Work out the finished part from the listing and answer in its coordinate system (mm). A direction names the side the tool comes from. Round coordinates to 2 decimals unless told otherwise and drop trailing zeros. Loops run counter-clockwise (first coordinate to the right, second up) from the corner with the lowest first, then second, coordinate; pieces in that order, holes last.
```python
from build123d import *

# Parameters (mm, degrees)
SKETCH1_W           = 8.89
SKETCH1_H           = 8.89
BOSS_EXTRUDE1_DEPTH = 5.334
SKETCH2_W           = 1.524
SKETCH2_H           = 8.89
CUT_EXTRUDE1_DEPTH  = 3.302
FILLET3_RADIUS      = 0.3683
FILLET3_LENGTH      = 8.89
FILLET4_RADIUS      = 0.254
FILLET4_LENGTH      = 8.89
FILLET5_RADIUS      = 0.254
FILLET5_LENGTH      = 8.89
FILLET6_RADIUS      = 0.254
FILLET6_LENGTH      = 8.89
FILLET7_RADIUS      = 0.2667
FILLET7_LENGTH      = 8.89


with BuildPart() as part:
    # Sketch1 → Boss-Extrude1 (new body)
    with BuildSketch(Plane(origin=(0, 0, 0), x_dir=(1, 0, 0), z_dir=(0, 1, 0))):
        Rectangle(SKETCH1_W, SKETCH1_H)
    extrude(amount=BOSS_EXTRUDE1_DEPTH)

    # Sketch2 → Cut-Extrude1 (cut)
    with BuildSketch(Plane(origin=(0, 5.334, 0), x_dir=(1, 0, 0), z_dir=(0, 1, 0))):
        with Locations((-3.1496, 0)):
            Rectangle(SKETCH2_W, SKETCH2_H)
        with Locations((-1.1176, 0)):
            Rectangle(SKETCH2_W, SKETCH2_H)
        with Locations((0.9144, 0)):
            Rectangle(SKETCH2_W, SKETCH2_H)
        with Locations((2.9464, 0)):
            Rectangle(SKETCH2_W, SKETCH2_H)
    extrude(amount=-CUT_EXTRUDE1_DEPTH, mode=Mode.SUBTRACT)

    # Fillet3: full round fillet: the end face becomes a half cylinder, R = half its width
    fillet3_face = Plane((4.0767, 5.334, 0), x_dir=(0, 0, -1), z_dir=(0, 1, 0))  # on the end face: x along it, z out of the body
    fillet3_slab = fillet3_face.offset(-FILLET3_RADIUS / 2) * Box(FILLET3_LENGTH, 2 * FILLET3_RADIUS, FILLET3_RADIUS, mode=Mode.PRIVATE)  # the body's end, R deep
    fillet3_round = Plane((4.0767, 4.9657, 0), x_dir=(0, 1, 0), z_dir=(0, 0, -1)) * Cylinder(FILLET3_RADIUS, FILLET3_LENGTH, mode=Mode.PRIVATE)  # its axis R under the face
    add(fillet3_slab - fillet3_round, mode=Mode.SUBTRACT)

    # Fillet4: full round fillet: the end face becomes a half cylinder, R = half its width
    fillet4_face = Plane((1.9304, 5.334, 0), x_dir=(0, 0, 1), z_dir=(0, 1, 0))  # on the end face: x along it, z out of the body
    fillet4_slab = fillet4_face.offset(-FILLET4_RADIUS / 2) * Box(FILLET4_LENGTH, 2 * FILLET4_RADIUS, FILLET4_RADIUS, mode=Mode.PRIVATE)  # the body's end, R deep
    fillet4_round = Plane((1.9304, 5.08, 0), x_dir=(0, 1, 0), z_dir=(0, 0, 1)) * Cylinder(FILLET4_RADIUS, FILLET4_LENGTH, mode=Mode.PRIVATE)  # its axis R under the face
    add(fillet4_slab - fillet4_round, mode=Mode.SUBTRACT)

    # Fillet5: full round fillet: the end face becomes a half cylinder, R = half its width
    fillet5_face = Plane((-0.1016, 5.334, 0), x_dir=(0, 0, 1), z_dir=(0, 1, 0))  # on the end face: x along it, z out of the body
    fillet5_slab = fillet5_face.offset(-FILLET5_RADIUS / 2) * Box(FILLET5_LENGTH, 2 * FILLET5_RADIUS, FILLET5_RADIUS, mode=Mode.PRIVATE)  # the body's end, R deep
    fillet5_round = Plane((-0.1016, 5.08, 0), x_dir=(0, 1, 0), z_dir=(0, 0, 1)) * Cylinder(FILLET5_RADIUS, FILLET5_LENGTH, mode=Mode.PRIVATE)  # its axis R under the face
    add(fillet5_slab - fillet5_round, mode=Mode.SUBTRACT)

    # Fillet6: full round fillet: the end face becomes a half cylinder, R = half its width
    fillet6_face = Plane((-2.1336, 5.334, 0), x_dir=(0, 0, 1), z_dir=(0, 1, 0))  # on the end face: x along it, z out of the body
    fillet6_slab = fillet6_face.offset(-FILLET6_RADIUS / 2) * Box(FILLET6_LENGTH, 2 * FILLET6_RADIUS, FILLET6_RADIUS, mode=Mode.PRIVATE)  # the body's end, R deep
    fillet6_round = Plane((-2.1336, 5.08, 0), x_dir=(0, 1, 0), z_dir=(0, 0, 1)) * Cylinder(FILLET6_RADIUS, FILLET6_LENGTH, mode=Mode.PRIVATE)  # its axis R under the face
    add(fillet6_slab - fillet6_round, mode=Mode.SUBTRACT)

    # Fillet7: full round fillet: the end face becomes a half cylinder, R = half its width
    fillet7_face = Plane((-4.1783, 5.334, 0), x_dir=(0, 0, 1), z_dir=(0, 1, 0))  # on the end face: x along it, z out of the body
    fillet7_slab = fillet7_face.offset(-FILLET7_RADIUS / 2) * Box(FILLET7_LENGTH, 2 * FILLET7_RADIUS, FILLET7_RADIUS, mode=Mode.PRIVATE)  # the body's end, R deep
    fillet7_round = Plane((-4.1783, 5.0673, 0), x_dir=(0, 1, 0), z_dir=(0, 0, 1)) * Cylinder(FILLET7_RADIUS, FILLET7_LENGTH, mode=Mode.PRIVATE)  # its axis R under the face
    add(fillet7_slab - fillet7_round, mode=Mode.SUBTRACT)


solid = part.part
```
1. Which of the six approach directions +Z, -Z, +X, -X, +Y, -Y give full straight-line access (tool end or side, diameter ignored) to faces 4 (the face through (-3.912, 4, 0)), 5 (the face through (0, 2, -4.445))?
Answer key:
face 4: +Z, -Z, +Y
face 5: -Z, +X, -X, +Y, -Y
2. Find section A-A (z = -1.25). Write down the section's boundary in (x, y) (3 decimals), then the cut area to 3 significant figures.
Answer key:
outline: (-4.445, 0) - (4.445, 0) - (4.445, 4.966) arc R0.368 ccw to (3.708, 4.966) - (3.708, 2.032) - (2.184, 2.032) - (2.184, 5.08) arc R0.254 ccw to (1.676, 5.08) - (1.676, 2.032) - (0.152, 2.032) - (0.152, 5.08) arc R0.254 ccw to (-0.356, 5.08) - (-0.356, 2.032) - (-1.88, 2.032) - (-1.88, 5.08) arc R0.254 ccw to (-2.388, 5.08) - (-2.388, 2.032) - (-3.912, 2.032) - (-3.912, 5.067) arc R0.267 ccw to (-4.445, 5.067) - close
area: 27.1 mm2
3. Consider probe 1 along X at (y, z) = (2.1, 2.25) (3 decimals); probe 2 along Y at (x, z) = (-3, -3). Determine where each line is inside the solid, lowest interval first.
Answer key:
probe 1: x = -4.445 to -3.912, -2.388 to -1.88, -0.356 to 0.152, 1.676 to 2.184, 3.708 to 4.445
probe 2: y = 0 to 2.03
4. Given pin 1 (1.7 mm diameter, centred on x = -1, z = -2, fed in from +Y), flat-ended and moving along its own axis, determine where the tip first touches the part or whether it passes through.
Answer key:
pin 1: stops at y = 5.33
5. Determine the mould class of faces 1 (the face through (-4.445, 2, 0)), 2 (the face through (0, 2, 4.445)), 3 (the face through (1.676, 4, 0)) for opening direction X: +X half, -X half, draft (parallel to the pull), parting line (faces both ways), or undercut.
Answer key:
face 1: -X half
face 2: draft
face 3: undercut
6. Find section B-B (x = 1). Write down the section's boundary in (y, z) (3 decimals).
Answer key:
outline: (0, -4.445) - (2.032, -4.445) - (2.032, 4.445) - (0, 4.445) - close
